Part model, mm, in its own coordinate system. Face numbers are marked on the shaded views. A direction names the side the tool comes from. Give positions to 0.01 mm unless a question says otherwise; leave off trailing zeros. Write each loop counter-clockwise with the first axis right and the second up, starting at its lowest first coordinate (ties: lowest second). Pieces come first, ordered by that corner, then holes. Notation, with made-up numbers: M 6,53 L 53,53 A27 ccw 53,72 Z; hole C -4,-24.75 d7. An arc over 180 degrees is marked long. Use a Markdown table: item, result.
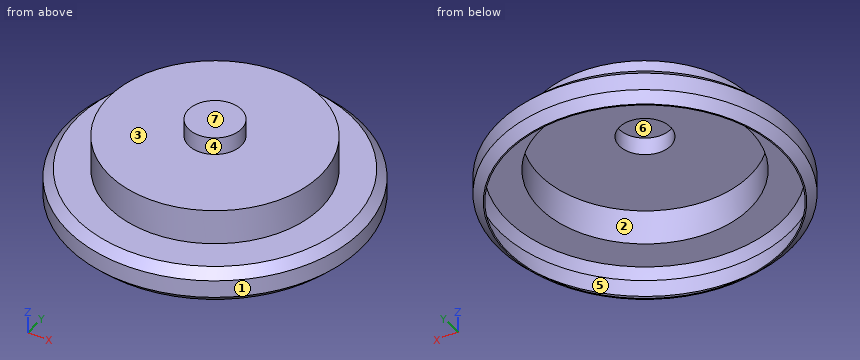
```python
from build123d import *

# Parameters (mm, degrees)
SKETCH1_R           = 76.2
BOSS_EXTRUDE1_DEPTH = 25.4
SKETCH2_R           = 19.05
BOSS_EXTRUDE2_DEPTH = 12.7
SKETCH3_R           = 105.541701
BOSS_EXTRUDE4_DEPTH = 25.4
CHAMFER1_SIZE       = 6.35
SHELL1_T            = -0.635


with BuildPart() as part:
    # Sketch1 → Boss-Extrude1 (new body)
    with BuildSketch(Plane.XY):
        Circle(SKETCH1_R)
    extrude(amount=BOSS_EXTRUDE1_DEPTH)

    # Sketch2 → Boss-Extrude2 (add)
    with BuildSketch(Plane.XY.offset(25.4)):
        Circle(SKETCH2_R)
    extrude(amount=BOSS_EXTRUDE2_DEPTH)

    # Sketch3 → Boss-Extrude4 (add)
    with BuildSketch(Plane(origin=(0, 0, 0), x_dir=(-1, 0, 0), z_dir=(0, 0, -1))):
        Circle(SKETCH3_R)
    extrude(amount=BOSS_EXTRUDE4_DEPTH)

    # Chamfer1
    chamfer1_edges = [part.edges().sort_by_distance(p)[0] for p in [
        (105.541701, 0, 0),
        (105.541701, 0, -25.4),
    ]]
    chamfer(chamfer1_edges, length=CHAMFER1_SIZE)

    # Shell1
    shell1_openings = [part.faces().sort_by_distance(p)[0] for p in [
        (-99.191701, 0, -25.4),
    ]]
    offset(amount=SHELL1_T, openings=shell1_openings, kind=Kind.INTERSECTION)


solid = part.part
```
1. Drop flat-ended pins along their axis: P1, Ø2, axis at x = -13.5, y = 31, coming from the +Z side; P2, Ø8, axis at x = -24, y = -8.5, coming from the -Z side (3 decimals); P3, Ø4, axis at y = 18, z = 11, coming from the +X side. Give the stop position or say it passes through.
Findings below:
| item | result |
|---|---|
| P1 | z = 25.4 |
| P2 | z = 24.765 |
| P3 | x = 74.5 |
2. Tool access for the marked faces 1, 2 and 3: list every direction of +Z, -Z, +X, -X, +Y, -Y with a clear straight run to the whole face (end or side of a thin tool).
Findings below:
| item | result |
|---|---|
| face 1 | +Z, -Z |
| face 2 | -Z |
| face 3 | +Z |
3. Two-plate mould, pull along X, no slides. Class the marked faces 4, 5, 6 and 7: released by +X, released by -X, zero draft, split by the parting line, or undercut.
Findings below:
| item | result |
|---|---|
| face 4 | split by the parting line |
| face 5 | undercut |
| face 6 | undercut |
| face 7 | zero draft |
4. Cut at A-A, the plane z = -12.5. Give the cut face in (x, y), then the cut area to 3 significant figures.
Findings below:
| item | result |
|---|---|
| outline | C 0,0 d211.08; hole C 0,0 d209.81 |
| area | 420 mm2 |
5. Cut at D-D, the plane z = 15.5. Give the cut face in (x, y) (3 decimals), then the cut area to 3 significant figures.
Findings below:
| item | result |
|---|---|
| outline | C 0,0 d152.4; hole C 0,0 d151.13 |
| area | 303 mm2 |
6. Drill centre lines: L1, parallel to Y at x = 0, z = -15; L2, parallel to Y at x = 0, z = 12.5 (3 decimals); L3, parallel to Z at x = -60, y = -21 (3 decimals). Where is each one in solid material? Low to high.
Findings below:
| item | result |
|---|---|
| L1 | -105.54 to -104.91, 104.91 to 105.54 |
| L2 | -76.2 to -75.565, 75.565 to 76.2 |
| L3 | 24.765 to 25.4 |
